Verification items for this drawing (mm, ordinates from the low corner). A direction names the side the tool comes from. Give positions to 0.01 mm unless a question says otherwise; leave off trailing zeros. Loops run counter-clockwise (first coordinate to the right, second up) from the corner with the lowest first, then second, coordinate; pieces in that order, holes last. Notation, with made-up numbers: (55.25, -8) -> (71.25, -8) arc R28 ccw to (71.25, 29) -> close; hole circle Ø6 at (18, 64.5). An arc over 180 degrees is marked (long way). Use one line per item in the form item = value. Start each with the question number.
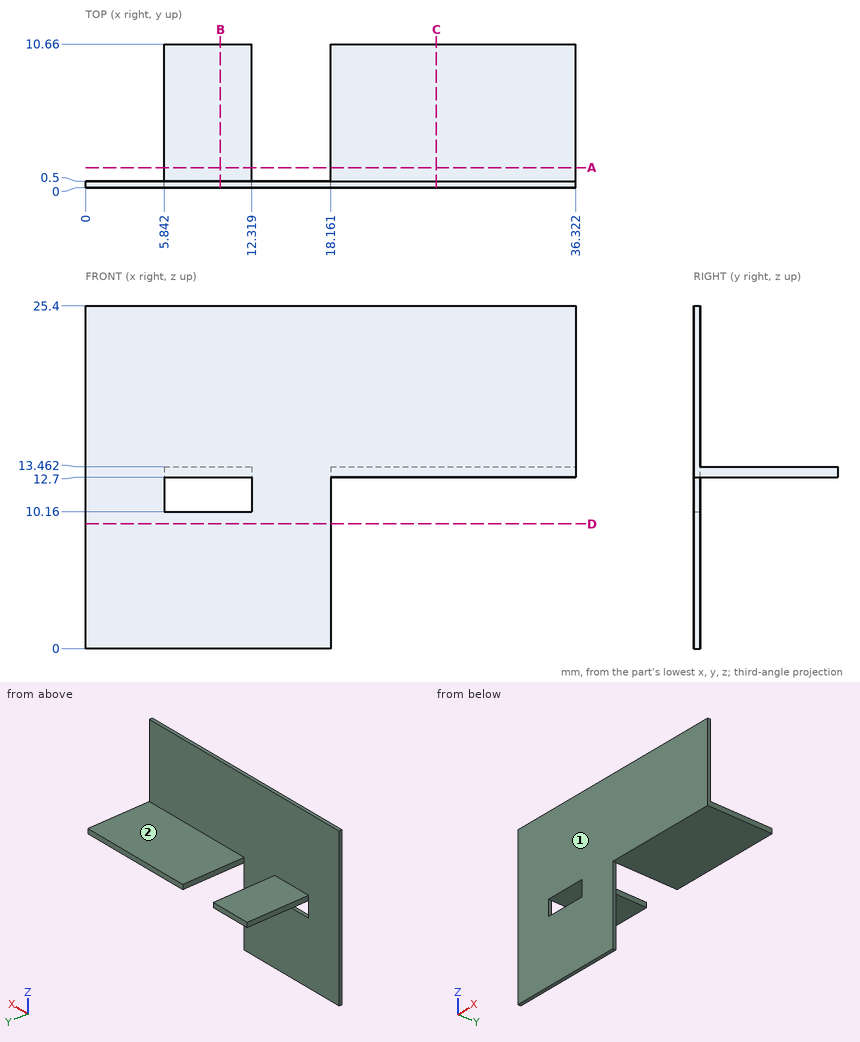
Item 1: Sectioned sample at C-C, the plane x = 26. Enter the section's corners in (y, z).
Item 2: Gauge pin test, flat ends, axial feed: pin 1 Ø2 at (x, z) = (13.5, 15) entering from +Y; pin 2 Ø0.8 at (y, z) = (5, 13) entering from -X; pin 3 Ø6 at (y, z) = (3, 6) entering from -X; pin 4 Ø3 at (x, y) = (23.5, 3.5) entering from -Z. Record the tip position at first contact, or that the pin passes through.
Item 3: Material ranges on line 1 (Z direction, x = 28, y = 4.5); line 2 (Y direction, x = 13, z = 8.5), recorded low to high.
Item 4: Tool access check on the marked faces 1 and 2. Record the directions out of +Z, -Z, +X, -X, +Y, -Y that give a thin tool (end or side, any length) a straight path to the whole face; none if there is none.
Item 5: Sectioned sample at A-A, the plane y = 1.5. Enter the section's corners in (x, z), and give its area (3 significant figures).
Item 6: Sectioned sample at B-B, the plane x = 10. Enter the section's corners in (y, z), and give its area (3 significant figures).
Item 7: Sectioned sample at D-D, the plane z = 9.25. Enter the section's corners in (x, y), and give its area (3 significant figures).
Outcome:
q1.outline = (0, 12.7) -> (10.66, 12.7) -> (10.66, 13.46) -> (0.5, 13.46) -> (0.5, 25.4) -> (0, 25.4) -> close
q2.pin_1 = 0.5
q2.pin_2 = 5.84
q2.pin_3 = 0
q2.pin_4 = 12.7
q3.line_1 = 12.7 to 13.46
q3.line_2 = 0 to 0.5
q4.face_1 = +Z, -Z, +X, -X, -Y
q4.face_2 = +Z, +X, -X, +Y
q5.outline = (5.84, 12.7) -> (12.32, 12.7) -> (12.32, 13.46) -> (5.84, 13.46) -> close; (18.16, 12.7) -> (36.32, 12.7) -> (36.32, 13.46) -> (18.16, 13.46) -> close
q5.area = 18.8 mm^2
q6.outline = (0, 0) -> (0.5, 0) -> (0.5, 10.16) -> (0, 10.16) -> close; (0, 12.7) -> (10.66, 12.7) -> (10.66, 13.46) -> (0.5, 13.46) -> (0.5, 25.4) -> (0, 25.4) -> close
q6.area = 19.2 mm^2
q7.outline = (0, 0) -> (18.16, 0) -> (18.16, 0.5) -> (0, 0.5) -> close
q7.area = 9.08 mm^2
